```python
from build123d import *

# Parameters (mm, degrees)
SKETCH1_R           = 4
SKETCH1_R_2         = 1.5
BOSS_EXTRUDE1_DEPTH = 8
CUT_EXTRUDE2_DEPTH  = 92.771795776
FILLET1_R           = 2
FILLET2_R           = 10


with BuildPart() as part:
    # Sketch1 → Boss-Extrude1 (new body)
    with BuildSketch(Plane(origin=(0, 0, 0), x_dir=(1, 0, 0), z_dir=(0, 1, 0))):
        Polygon((0, 0), (0, -80), (44.25, -80), (44.25, -64), (12, -64), (12, -16), (44.25, -16), (44.25, 0), align=None)
        with Locations(Location((39, -8, 0), (0, 0, 270))):
            Circle(SKETCH1_R, mode=Mode.SUBTRACT)
        with Locations(Location((39, -72, 0), (0, 0, 90))):
            Circle(SKETCH1_R, mode=Mode.SUBTRACT)
        with Locations(Location((24, -8, 0), (0, 0, 270))):
            Circle(SKETCH1_R_2, mode=Mode.SUBTRACT)
        with Locations(Location((9, -8, 0), (0, 0, 270))):
            Circle(SKETCH1_R_2, mode=Mode.SUBTRACT)
        with Locations(Location((24, -72, 0), (0, 0, 90))):
            Circle(SKETCH1_R_2, mode=Mode.SUBTRACT)
        with Locations(Location((9, -72, 0), (0, 0, 90))):
            Circle(SKETCH1_R_2, mode=Mode.SUBTRACT)
    extrude(amount=BOSS_EXTRUDE1_DEPTH)

    # Sketch4 → Cut-Extrude2 (cut, through all)
    with BuildSketch(Plane(origin=(0, 8, 0), x_dir=(1, 0, 0), z_dir=(0, 1, 0))):
        with BuildLine():
            Line((39, -7.5), (44.25, -7.5))
            ThreePointArc((44.25, -7.5), (44.75, -8), (44.25, -8.5))
            Line((44.25, -8.5), (39, -8.5))
            ThreePointArc((39, -8.5), (38.5, -8), (39, -7.5))
        make_face()
        with BuildLine():
            Line((39, -71.5), (44.25, -71.5))
            ThreePointArc((44.25, -71.5), (44.75, -72), (44.25, -72.5))
            Line((44.25, -72.5), (39, -72.5))
            ThreePointArc((39, -72.5), (38.5, -72), (39, -71.5))
        make_face()
    extrude(amount=-CUT_EXTRUDE2_DEPTH, mode=Mode.SUBTRACT)

    # Fillet1
    fillet1_edges = [part.edges().sort_by_distance(p)[0] for p in [
        (44.25, 4, 0),
        (44.25, 4, 16),
        (44.25, 4, 64),
        (44.25, 4, 80),
    ]]
    fillet(fillet1_edges, radius=FILLET1_R)

    # Fillet2
    fillet2_edges = [part.edges().sort_by_distance(p)[0] for p in [
        (12, 4, 16),
        (12, 4, 64),
    ]]
    fillet(fillet2_edges, radius=FILLET2_R)


solid = part.part
```
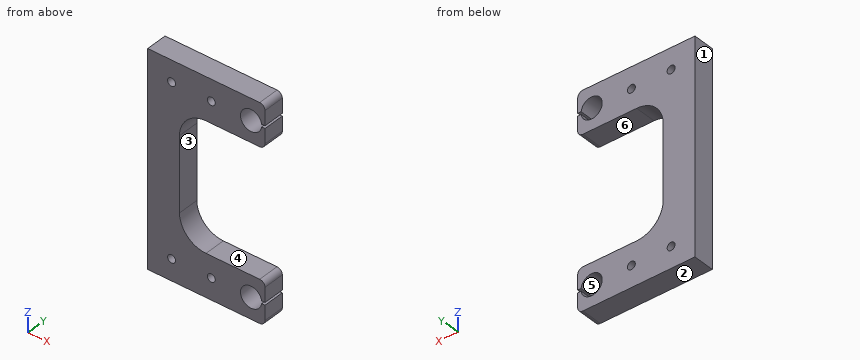
Input: part model. Units: mm. Frame: model coordinates. Face numbers are marked on the shaded views. A direction names the side the tool comes from. Coordinates: 2 decimals unless noted, no trailing zeros. Write each loop counter-clockwise with the first axis right and the second up, starting at its lowest first coordinate (ties: lowest second). Pieces come first, ordered by that corner, then holes. Notation, with made-up numbers: M 45.25,47 L 72.25,47 A18 ccw 72.25,67 Z; hole C -3,58 d9. An arc over 180 degrees is marked long. Use one line per item in the form item = value.
Q1. Section B-B (y = 1.75). Return loops of the section in (x, z), plus the area to 3 significant figures.
Answer below:
outline = M 0,0 L 42.25,0 A2 ccw 44.25,2 L 44.25,7.5 L 42.97,7.5 A4 cw long 42.97,8.5 L 44.25,8.5 L 44.25,14 A2 ccw 42.25,16 L 22,16 A10 cw 12,26 L 12,54 A10 cw 22,64 L 42.25,64 A2 ccw 44.25,66 L 44.25,71.5 L 42.97,71.5 A4 cw long 42.97,72.5 L 44.25,72.5 L 44.25,78 A2 ccw 42.25,80 L 0,80 Z; hole C 9,8 d3; hole C 9,72 d3; hole C 24,8 d3; hole C 24,72 d3
area = 1,900 mm²
Q2. Section D-D (x = 9). Return loops of the section in (y, z), plus the area to 3 significant figures.
Answer below:
outline = M 0,0 L 8,0 L 8,6.5 L 0,6.5 Z; M 0,9.5 L 8,9.5 L 8,70.5 L 0,70.5 Z; M 0,73.5 L 8,73.5 L 8,80 L 0,80 Z
area = 592 mm²
Q3. Section A-A (x = 27.5). Return loops of the section in (y, z).
Answer below:
outline = M 0,0 L 8,0 L 8,16 L 0,16 Z; M 0,64 L 8,64 L 8,80 L 0,80 Z
Q4. Set-up query: the marked faces 5 and 6. Return all of +Z, -Z, +X, -X, +Y, -Y with unobstructed straight access to the full face (end or side cutting, diameter ignored); none if empty.
Answer below:
face_5 = +Y, -Y
face_6 = +X, +Y, -Y
Q5. First-contact query: pin 1 (0.6 mm diameter, centred on x = 43.5, y = 4.5, fed in from -Z); pin 2 (1 mm diameter, centred on y = 5.5, z = 38.5, fed in from +X). Flat tips, straight axial feed; report the tip coordinate or a pass-through.
Answer below:
pin_1 = 0.24
pin_2 = 12
Q6. Draft query along Z for the marked faces 1, 2, 3 and 4. Return one class per face: released by +Z, released by -Z, zero draft, split by the parting line, or undercut.
Answer below:
face_1 = zero draft
face_2 = released by -Z
face_3 = undercut
face_4 = undercut
Q7. Section C-C (x = 39). Return loops of the section in (y, z).
Answer below:
outline = M 0,0 L 8,0 L 8,4 L 0,4 Z; M 0,12 L 8,12 L 8,16 L 0,16 Z; M 0,64 L 8,64 L 8,68 L 0,68 Z; M 0,76 L 8,76 L 8,80 L 0,80 Z
Q8. Material intervals for probe 1 along Z at (x, y) = (28, 7.5); probe 2 along Z at (x, y) = (39, 5); probe 3 along Z at (x, y) = (40, 4.25), sorted ascending. Write a range as from..to.
Answer below:
probe_1 = 0..16, 64..80
probe_2 = 0..4, 12..16, 64..68, 76..80
probe_3 = 0..4.13, 11.87..16, 64..68.13, 75.87..80
